from build123d import *

# Parameters (mm, degrees)
CYLINDER121_R          = 1.8
CYLINDER121_DEPTH      = 34
CYLINDER121_ROLL_ANGLE = 90
PAD057_DEPTH           = 20
CYLINDER118_R          = 1.8
CYLINDER118_DEPTH      = 34
CYLINDER118_ROLL_ANGLE = 90
CYLINDER117_R          = 1.8
CYLINDER117_DEPTH      = 34
CYLINDER117_ROLL_ANGLE = 90
CYLINDER120_R          = 1.8
CYLINDER120_DEPTH      = 34
CYLINDER120_ROLL_ANGLE = 90
CYLINDER119_R          = 1.8
CYLINDER119_DEPTH      = 34
CYLINDER119_ROLL_ANGLE = 90
BOX059_W               = 50
BOX059_H               = 4
BOX059_DEPTH           = 52
FILLET054_R            = 5


with BuildPart() as cilindro075:
    # Cylinder121 → Cylinder121 (new body)
    with BuildSketch(Plane.XY):
        Circle(CYLINDER121_R)
    extrude(amount=CYLINDER121_DEPTH)


with BuildPart() as cilindro075_1:
    # Cylinder121 roll: moved
    add(cilindro075.part.rotate(Axis((0, 0, 0), (1, 0, 0)), CYLINDER121_ROLL_ANGLE))


with BuildPart() as cilindro075_2:
    # Cylinder121 placement: moved
    add(cilindro075_1.part.moved(Location((33, -26, 85))))


with BuildPart() as cut139:
    # Sketch064 → Pad057 (new body)
    with BuildSketch(Plane(origin=(2, 0, 75), x_dir=(1, 0, 0), z_dir=(0, 0, 1))):
        with BuildLine():
            ThreePointArc((17.453972, -22.45432), (31.040886, -36.073109), (44.6278, -22.45432))
            Line((17.453972, -22.45432), (44.6278, -22.45432))
        make_face()
        Polygon((26.782288, -29.812588), (29.287536, -32.286525), (32.808351, -32.264384), (35.282288, -29.759136), (35.260147, -26.238321), (32.754899, -23.764384), (29.234084, -23.786525), (26.760147, -26.291773), align=None, mode=Mode.SUBTRACT)
    extrude(amount=PAD057_DEPTH)

    # Cut139: cut Cilindro075
    add(cilindro075_2.part, mode=Mode.SUBTRACT)


with BuildPart() as cut139_1:
    # Cut139 placement: moved
    add(cut139.part.moved(Location((0, -0.2, 0))))


with BuildPart() as cilindro072:
    # Cylinder118 → Cylinder118 (new body)
    with BuildSketch(Plane.XY):
        Circle(CYLINDER118_R)
    extrude(amount=CYLINDER118_DEPTH)


with BuildPart() as cilindro072_1:
    # Cylinder118 roll: moved
    add(cilindro072.part.rotate(Axis((0, 0, 0), (1, 0, 0)), CYLINDER118_ROLL_ANGLE))


with BuildPart() as cilindro072_2:
    # Cylinder118 placement: moved
    add(cilindro072_1.part.moved(Location((16, -10, 63))))


with BuildPart() as fusion066:
    # Cylinder117 → Cylinder117 (new body)
    with BuildSketch(Plane.XY):
        Circle(CYLINDER117_R)
    extrude(amount=CYLINDER117_DEPTH)


with BuildPart() as fusion066_1:
    # Cylinder117 roll: moved
    add(fusion066.part.rotate(Axis((0, 0, 0), (1, 0, 0)), CYLINDER117_ROLL_ANGLE))


with BuildPart() as fusion066_2:
    # Cylinder117 placement: moved
    add(fusion066_1.part.moved(Location((50, -10, 63))))

    # Fusion066: union Cilindro072
    add(cilindro072_2.part)


with BuildPart() as cilindro074:
    # Cylinder120 → Cylinder120 (new body)
    with BuildSketch(Plane.XY):
        Circle(CYLINDER120_R)
    extrude(amount=CYLINDER120_DEPTH)


with BuildPart() as cilindro074_1:
    # Cylinder120 roll: moved
    add(cilindro074.part.rotate(Axis((0, 0, 0), (1, 0, 0)), CYLINDER120_ROLL_ANGLE))


with BuildPart() as cilindro074_2:
    # Cylinder120 placement: moved
    add(cilindro074_1.part.moved(Location((16, -10, 63))))


with BuildPart() as fusion068:
    # Cylinder119 → Cylinder119 (new body)
    with BuildSketch(Plane.XY):
        Circle(CYLINDER119_R)
    extrude(amount=CYLINDER119_DEPTH)


with BuildPart() as fusion068_1:
    # Cylinder119 roll: moved
    add(fusion068.part.rotate(Axis((0, 0, 0), (1, 0, 0)), CYLINDER119_ROLL_ANGLE))


with BuildPart() as fusion068_2:
    # Cylinder119 placement: moved
    add(fusion068_1.part.moved(Location((50, -10, 63))))

    # Fusion067: union Cilindro074
    add(cilindro074_2.part)


with BuildPart() as fusion068_3:
    # Fusion067 placement: moved
    add(fusion068_2.part.moved(Location((0, 0, 43))))

    # Fusion068: union Fusion066
    add(fusion066_2.part)


with BuildPart() as lapis_holder:
    # Box059 → Box059 (new body)
    with BuildSketch(Plane(origin=(8, -23, 59), x_dir=(1, 0, 0), z_dir=(0, 0, 1))):
        with Locations((25, 2)):
            Rectangle(BOX059_W, BOX059_H)
    extrude(amount=BOX059_DEPTH)

    # Cut138: cut Fusion068
    add(fusion068_3.part, mode=Mode.SUBTRACT)

    # Fusion069: union Cut139
    add(cut139_1.part)

    # Fillet054
    fillet054_edges = [lapis_holder.edges().sort_by_distance(p)[0] for p in [
        (8, -21, 111),
        (8, -21, 59),
        (58, -21, 111),
        (58, -21, 59),
    ]]
    fillet(fillet054_edges, radius=FILLET054_R)


solid = lapis_holder.part
Can you work these out from the model? Positions are in its coordinate system, mm. A direction names the side the tool comes from. Round coordinates to 2 decimals unless told otherwise and drop trailing zeros. Loops run counter-clockwise (first coordinate to the right, second up) from the corner with the lowest first, then second, coordinate; pieces in that order, holes last. Notation, with made-up numbers: (60.5, -37) - (110.5, -37) arc R27 cw to (110.5, -4) - close; hole circle Ø9 at (58, -22). An arc over 180 degrees is marked (long way). Use CSV: the item, a comma, the result in double quotes. Start each with the question number.
1) If we section it at A-A on x = 50: Write out the boundary of the cut face in (y, z), plus the area to 3 significant figures.
2) If we section it at C-C on y = -25.5: Write out the boundary of the cut face in (x, z).
3) Please list where these lines run through material, in increasing order: probe 1 along Z at (x, y) = (16, -21.6); probe 2 along Y at (x, z) = (33.5, 88); probe 3 along X at (y, z) = (-19.95, 63). Write a range as [from, to].
4) For faces 5 (the cylindrical face through (34.663, -34.302, 84.311)), 6 (the cylindrical face through (56, -21, 110)), 7 (the flat face through (30.014, -25.222, 84.86)), which set-ups out of +Z, -Z, +X, -X, +Y, -Y let a thin tool reach every point of the face, with its end or its side?
5) If we section it at B-B on z = 63: Write out the boundary of the cut face in (x, y).
6) For pin 1 Ø4.5 at (x, z) = (50, 106) entering from +Y; pin 2 Ø1 at (x, y) = (21.5, -24) entering from +Z; pin 3 Ø1 at (y, z) = (-27.5, 75.5) entering from -X; pin 4 Ø4 at (x, z) = (50, 63) entering from -Y, each with a flat end and sliding along its axis, tell me the tip position at first contact or that it passes through.
7) We'd pull the mould along Z, two halves only. Please class faces 1 (the cylindrical face through (49.766, -20.972, 64.785)), 2 (the cylindrical face through (9, -21, 109)), 3 (the flat face through (8, -21, 85)), 4 (the flat face through (30, -25, 75)): released by +Z, released by -Z, zero draft, split by the parting line, or undercut.
Geometry results:
1,outline,"(-23, 59) - (-19, 59) - (-19, 61.2) - (-23, 61.2) - close; (-23, 64.8) - (-19, 64.8) - (-19, 104.2) - (-23, 104.2) - close; (-23, 107.8) - (-19, 107.8) - (-19, 111) - (-23, 111) - close"
1,area,"179 mm2"
2,outline,"(19.75, 75) - (29.74, 75) - (29.74, 95) - (19.75, 95) - close; (36.31, 75) - (46.33, 75) - (46.33, 95) - (36.31, 95) - close"
3,probe 1,"z = [59, 61.2], [64.8, 104.2], [107.8, 111]"
3,probe 2,"y = [-36.27, -32.47], [-23.97, -19]"
3,probe 3,"x = [8.1, 14.2], [17.8, 48.2], [51.8, 57.9]"
4,face 5,"-Y"
4,face 6,"+Z, +X, +Y, -Y"
4,face 7,"+Z, -Z"
5,outline,"(8.1, -23) - (14.2, -23) - (14.2, -19) - (8.1, -19) - close; (17.8, -23) - (48.2, -23) - (48.2, -19) - (17.8, -19) - close; (51.8, -23) - (57.9, -23) - (57.9, -19) - (51.8, -19) - close"
6,pin 1,"stops at y = -19"
6,pin 2,"stops at z = 95"
6,pin 3,"stops at x = 20.16"
6,pin 4,"stops at y = -23"
7,face 1,"undercut"
7,face 2,"released by +Z"
7,face 3,"zero draft"
7,face 4,"released by -Z"
